from build123d import *

# Parameters (mm, degrees)
BOSS_EXTRUDE1_DEPTH = 12.6
SKETCH2_R           = 1.9
BOSS_EXTRUDE2_DEPTH = 3.1


with BuildPart() as part:
    # Sketch1 → Boss-Extrude1 (new body)
    with BuildSketch(Plane.XY):
        with BuildLine():
            Line((-0.937749967, 2.425), (0.937749967, 2.425))
            ThreePointArc((0.937749967, 2.425), (2.6, 0), (0.937749967, -2.425))
            Line((0.937749967, -2.425), (-0.937749967, -2.425))
            ThreePointArc((-0.937749967, -2.425), (-2.6, 0), (-0.937749967, 2.425))
        make_face()
    extrude(amount=BOSS_EXTRUDE1_DEPTH)

    # Sketch2 → Loft1 section 0
    with BuildSketch(Plane.XY.offset(14)):
        Circle(SKETCH2_R)
    # Sketch3 → Loft1 section 1
    with BuildSketch(Plane.XY.offset(12.6)):
        with BuildLine():
            Line((-0.937749967, -2.425), (0.937749967, -2.425))
            ThreePointArc((0.937749967, -2.425), (2.6, 0), (0.937749967, 2.425))
            Line((0.937749967, 2.425), (-0.937749967, 2.425))
            ThreePointArc((-0.937749967, 2.425), (-2.6, 0), (-0.937749967, -2.425))
        make_face()
    loft()

    # Sketch4 → Boss-Extrude2 (add)
    with BuildSketch(Plane.XY.offset(14)):
        with BuildLine():
            ThreePointArc((0.685278822, 1.772115385), (0, 1.9), (-0.685278822, 1.772115385))
            ThreePointArc((-0.685278822, 1.772115385), (-1.9, 0), (-0.685278822, -1.772115385))
            ThreePointArc((-0.685278822, -1.772115385), (0, -1.9), (0.685278822, -1.772115385))
            ThreePointArc((0.685278822, -1.772115385), (1.9, 0), (0.685278822, 1.772115385))
        make_face()
    extrude(amount=BOSS_EXTRUDE2_DEPTH)


solid = part.part
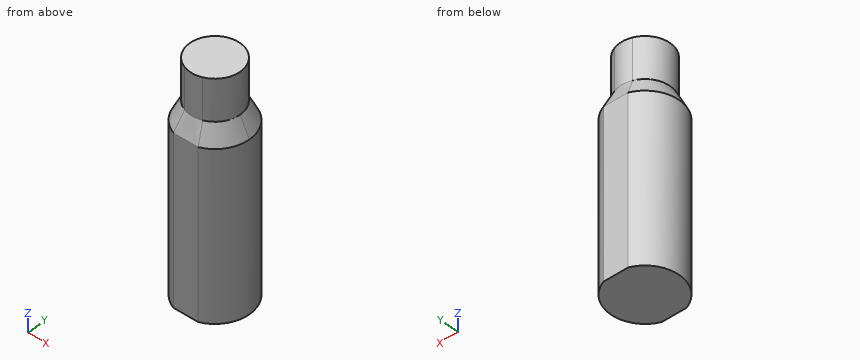
The listing builds one solid part. Answer for the finished solid, in the listing's coordinates (mm). Give positions to 0.01 mm unless a question says otherwise; leave off trailing zeros. Loops run counter-clockwise (first coordinate to the right, second up) from the corner with the lowest first, then second, coordinate; pieces in that order, holes last. Notation, with made-up numbers: M 12.5,22 L 63.5,22 A26 cw 63.5,58 Z; hole C 68.5,5.5 d3. An arc over 180 degrees is marked long. Answer as CSV lines item,"result".
Item 1: The part is cut by section A-A (z = 5.25). Give the vertices of the cut face in (x, y) (3 decimals).
Values follow:
outline,"M -0.938,-2.425 L 0.938,-2.425 A2.6 ccw 0.938,2.425 L -0.938,2.425 A2.6 ccw Z"
Item 2: Straight lines are drawn through the part: line 1 along Z through (x, y) = (2, -1.2); line 2 along X through (y, z) = (0.65, 4.25); line 3 along Z through (x, y) = (-1.9, 1.65). For each, find the intervals that lie inside material, in ascending order. Write a range as [from, to].
Values follow:
line 1,"z = [0, 13.14]"
line 2,"x = [-2.52, 2.52]"
line 3,"z = [0, 12.77]"
Item 3: Given pin 1 Ø2 at (x, y) = (2, 1.5) entering from +Z, flat-ended and moving along its own axis, determine where the tip first touches the part or whether it passes through.
Values follow:
pin 1,"stops at z = 17.1"
